The listing builds one solid part. Answer for the finished solid, in the listing's coordinates (mm). Coordinates: 2 decimals unless noted, no trailing zeros. Order: outer loops, then holes, each group sorted by start corner. A loop starts at its lowest first (then second) coordinate and runs counter-clockwise, first axis right, second up. Notation, with made-up numbers: M 0,25.5 L 37,25.5 A19 ccw 37,56.5 Z; hole C 89,53.25 d4. An arc over 180 degrees is marked long. One line per item, written item: value. Start each with the question number.
Q1. The part is cut by section B-B on x = 15. Give the vertices of the cut face in (y, z), then the cut area to 3 significant figures.
Q2. The part is cut by section C-C on z = -3. Give the vertices of the cut face in (x, y), then the cut area to 3 significant figures.
Q3. Straight lines are drawn through the part: line 1 along Y through (x, z) = (42.7, -4.6); line 2 along Y through (x, z) = (98.4, 4.45); line 3 along Y through (x, z) = (45.5, 3.5). For each, find the intervals that lie inside material, in ascending order. Write a range as [from, to].
Q4. Each of these flat-tipped pins is pushed along its axis until it touches: pin 1 Ø2.5 at (x, y) = (98.4, -5) entering from +Z; pin 2 Ø3.5 at (x, y) = (15, 5) entering from -Z. Where does it stop, or does it pass through?
Q5. The part is cut by section A-A on y = -2. Give the vertices of the cut face in (x, z).
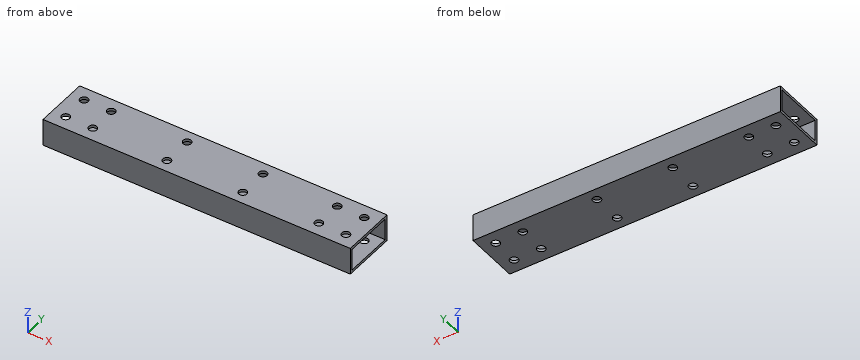
```python
from build123d import *

# Parameters (mm, degrees)
SKETCH_11_W                = 20
SKETCH_11_H                = 10
SKETCH_11_W_2              = 18
SKETCH_11_H_2              = 8
JIQIRENDUI_20X10X1_1_DEPTH = 113.4
SKETCH_12_R                = 1.5
CUT_EXTRUDE_1_DEPTH        = 10
SKETCH_13_R                = 1.5
CUT_EXTRUDE_2_DEPTH        = 115.278431911


with BuildPart() as part:
    # 草图11 → Jiqirendui 20X10X1(1) (new body)
    with BuildSketch(Plane.YZ):
        Rectangle(SKETCH_11_W, SKETCH_11_H)
        Rectangle(SKETCH_11_W_2, SKETCH_11_H_2, mode=Mode.SUBTRACT)
    extrude(amount=JIQIRENDUI_20X10X1_1_DEPTH)

    # 草图12 → 切除-拉伸1 (cut)
    with BuildSketch(Plane.XY.offset(5)):
        with Locations((15, 5)):
            Circle(SKETCH_12_R)
        with Locations((5, 5)):
            Circle(SKETCH_12_R)
        with Locations((15, -5)):
            Circle(SKETCH_12_R)
        with Locations((5, -5)):
            Circle(SKETCH_12_R)
        with Locations((108.4, -5)):
            Circle(SKETCH_12_R)
        with Locations((108.4, 5)):
            Circle(SKETCH_12_R)
        with Locations((98.4, 5)):
            Circle(SKETCH_12_R)
        with Locations((98.4, -5)):
            Circle(SKETCH_12_R)
    extrude(amount=-CUT_EXTRUDE_1_DEPTH, mode=Mode.SUBTRACT)

    # 草图13 → 切除-拉伸2 (cut, through all)
    with BuildSketch(Plane.XY.offset(5)):
        with Locations((42.7, 5.5)):
            Circle(SKETCH_13_R)
        with Locations(Location((70.7, 5.5, 0), (0, 0, 90))):
            Circle(SKETCH_13_R)
        with Locations((70.7, -5.5)):
            Circle(SKETCH_13_R)
        with Locations(Location((42.7, -5.5, 0), (0, 0, 90))):
            Circle(SKETCH_13_R)
    extrude(amount=-CUT_EXTRUDE_2_DEPTH, mode=Mode.SUBTRACT)


solid = part.part
```
Output:
1. outline: M -10,-5 L -6.5,-5 L -6.5,-4 L -9,-4 L -9,4 L -6.5,4 L -6.5,5 L -10,5 Z; M -3.5,-5 L 3.5,-5 L 3.5,-4 L -3.5,-4 Z; M -3.5,4 L 3.5,4 L 3.5,5 L -3.5,5 Z; M 6.5,-5 L 10,-5 L 10,5 L 6.5,5 L 6.5,4 L 9,4 L 9,-4 L 6.5,-4 Z
1. area: 44.0 mm^2
2. outline: M 0,-10 L 113.4,-10 L 113.4,-9 L 0,-9 Z; M 0,9 L 113.4,9 L 113.4,10 L 0,10 Z
2. area: 227 mm^2
3. line 1: y = [-10, -7], [-4, 4], [7, 10]
3. line 2: y = [-10, -6.5], [-3.5, 3.5], [6.5, 10]
3. line 3: y = [-10, -9], [9, 10]
4. pin 1: passes through
4. pin 2: stops at z = -5
5. outline: M 0,-5 L 113.4,-5 L 113.4,-4 L 0,-4 Z; M 0,4 L 113.4,4 L 113.4,5 L 0,5 Z
